For this review, use the dimensioned drawing (mm, ordinates from the lowest corner) and the shaded views. Round coordinates to 2 decimals unless told otherwise and drop trailing zeros. Write each loop counter-clockwise with the first axis right and the second up, starting at its lowest first coordinate (ties: lowest second). Pieces come first, ordered by that corner, then holes.
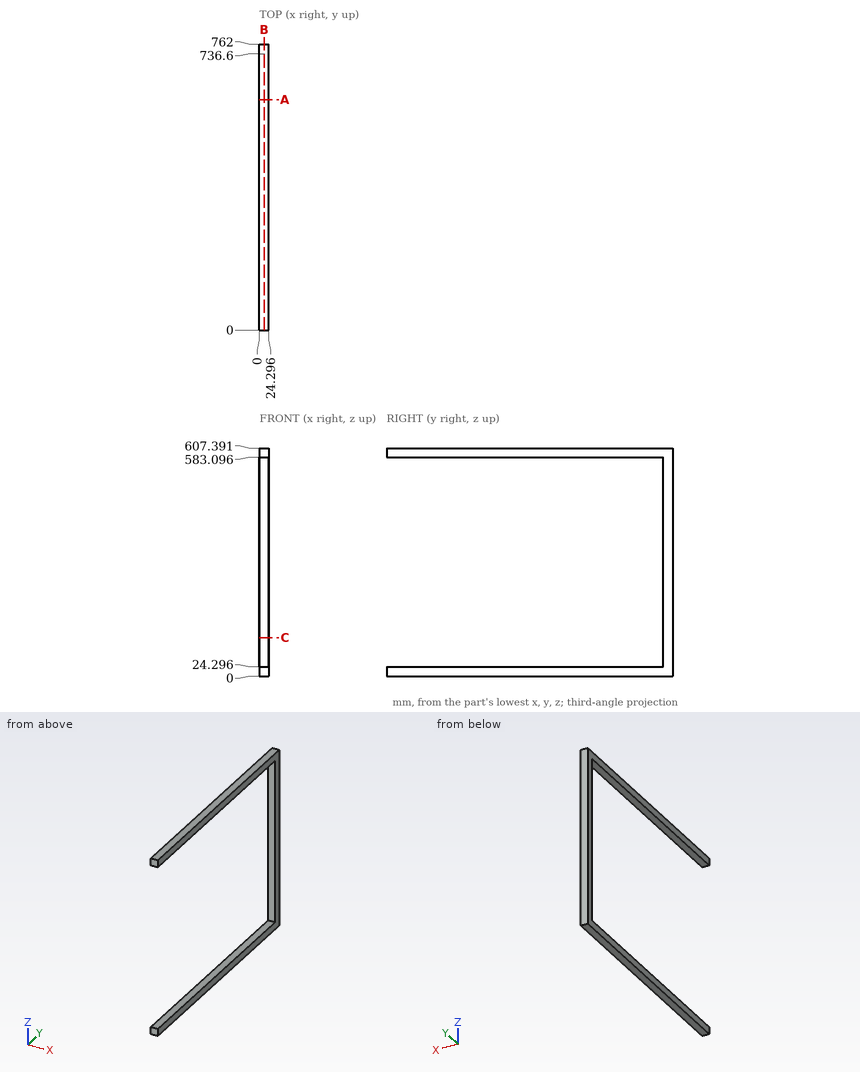
1) Add section C-C on z = 102.5. State the section outline as (x, y) points (1 decimal), and give its area (3 significant figures).
2) For line 1 along Z through (x, y) = (21.25, 87) (1 decimal); line 2 along Y through (x, z) = (17.5, 342), list the stretches that pass through material, from the lowest coordinate up.
3) For P1, Ø12, axis at x = 9.5, z = 201, coming from the -Y side, flat-tipped, find the tip position at first contact; note if it passes through.
4) Add section A-A on y = 614. State the section outline as (x, z) points (1 decimal).
5) Add section B-B on x = 12.75. State the section outline as (y, z) points (1 decimal).
Computed:
1. outline: (0, 736.6) - (24.3, 736.6) - (24.3, 762) - (0, 762) - close
1. area: 617 mm2
2. line 1: z = 0 to 24.3, 583.1 to 607.4
2. line 2: y = 736.6 to 762
3. P1: stops at y = 736.6
4. outline: (0, 0) - (24.3, 0) - (24.3, 24.3) - (0, 24.3) - close; (0, 583.1) - (24.3, 583.1) - (24.3, 607.4) - (0, 607.4) - close
5. outline: (0, 0) - (762, 0) - (762, 607.4) - (0, 607.4) - (0, 583.1) - (736.6, 583.1) - (736.6, 24.3) - (0, 24.3) - close
